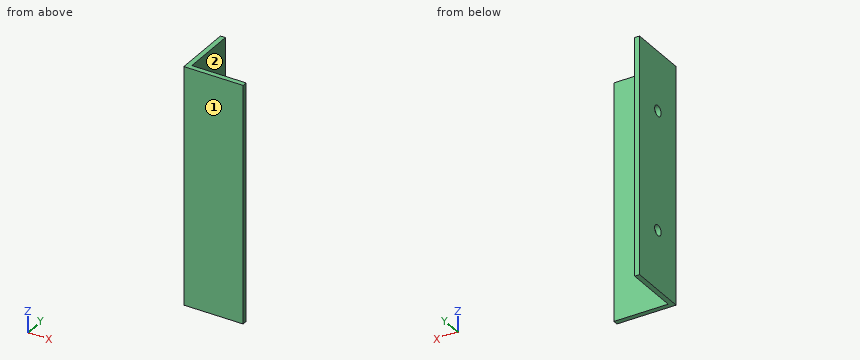
from build123d import *

# Parameters (mm, degrees)
BOSS_EXTRUDE1_DEPTH     = 152.4
F_1_4_CLEARANCE_HOLE1_D = 6.7564


with BuildPart() as part:
    # Sketch1 → Boss-Extrude1 (new body)
    with BuildSketch(Plane.XY):
        Polygon((0, 0), (0, 38.1), (3.175, 38.1), (3.175, 3.175), (38.1, 3.175), (38.1, 0), align=None)
    extrude(amount=BOSS_EXTRUDE1_DEPTH)

    # 1/4 Clearance Hole1 (through all)
    with Locations(Plane.ZY):
        with Locations((38.1, 19.05), (114.3, 19.05)):
            Hole(F_1_4_CLEARANCE_HOLE1_D / 2)


solid = part.part
Model file for the job. Use its own axes, mm. Face numbers are marked on the shaded views. A direction names the side the tool comes from. Round coordinates to 2 decimals unless told otherwise and drop trailing zeros. Order: outer loops, then holes, each group sorted by start corner. A loop starts at its lowest first (then second) coordinate and runs counter-clockwise, first axis right, second up. Notation, with made-up numbers: M 75,-11.5 L 130,-11.5 A28 ccw 130,20.5 Z; hole C -34.75,-15 d4. An arc over 180 degrees is marked long. Write each question's results on one line, items separated by ' | '. Start each with the question number.
(1) Saw through at D-D, the plane x = 11. Give the cut face in (y, z) (3 decimals), then the cut area to 3 significant figures.
(2) Which spindle directions (+Z, -Z, +X, -X, +Y, -Y) get a long thin tool onto all of the face, cutting with end or side? Do the marked faces 1 and 2. Say none if no direction does.
(3) Saw through at C-C, the plane z = 62.5. Give the cut face in (x, y) (3 decimals), then the cut area to 3 significant figures.
(4) Saw through at A-A, the plane z = 114.3. Give the cut face in (x, y) (3 decimals).
(5) Drop flat-ended pins along their axis: pin 1 (1 mm diameter, centred on x = 14.5, z = 68.5, fed in from +Y) (3 decimals); pin 2 (4 mm diameter, centred on y = 8.5, z = 111, fed in from +X) (3 decimals); pin 3 (6 mm diameter, centred on x = 30.5, z = 86, fed in from -Y). Give the stop position or say it passes through.
(6) Saw through at B-B, the plane y = 19.05. Give the cut face in (x, z) (3 decimals).
(7) Probe probe 1 along Z at (x, y) = (1, 19); probe 2 along Y at (x, z) = (2.5, 114.3); probe 3 along Z at (x, y) = (2, 17). List the from-to ranges inside material, lowest first. Write a range as from..to.
Established:
1) outline: M 0,0 L 3.175,0 L 3.175,152.4 L 0,152.4 Z | area: 484 mm^2
2) face 1: +Z, -Z, +X, -X, -Y | face 2: +Z, -Z, +X, +Y
3) outline: M 0,0 L 38.1,0 L 38.1,3.175 L 3.175,3.175 L 3.175,38.1 L 0,38.1 Z | area: 232 mm^2
4) outline: M 0,0 L 38.1,0 L 38.1,3.175 L 3.175,3.175 L 3.175,15.672 L 0,15.672 Z; M 0,22.428 L 3.175,22.428 L 3.175,38.1 L 0,38.1 Z
5) pin 1: stops at y = 3.175 | pin 2: stops at x = 3.175 | pin 3: stops at y = 0
6) outline: M 0,0 L 3.175,0 L 3.175,34.722 L 0,34.722 Z; M 0,41.478 L 3.175,41.478 L 3.175,110.922 L 0,110.922 Z; M 0,117.678 L 3.175,117.678 L 3.175,152.4 L 0,152.4 Z
7) probe 1: z = 0..34.72, 41.48..110.92, 117.68..152.4 | probe 2: y = 0..15.67, 22.43..38.1 | probe 3: z = 0..35.41, 40.79..111.61, 116.99..152.4
